Study the drawing (mm; zero at the part's minimum x, y, z) and answer. A direction names the side the tool comes from. Round coordinates to 2 decimals unless told otherwise and drop trailing zeros. Write each loop counter-clockwise with the first axis right and the second up, starting at its lowest first coordinate (ties: lowest second). Pieces come first, ordered by that corner, then holes. Notation, with made-up numbers: M 58.25,-30 L 78.25,-30 A21 ccw 78.25,-11 Z; hole C 52.5,54 d1. An arc over 180 degrees is marked long. Write each question's results on one line, items separated by ' | '.
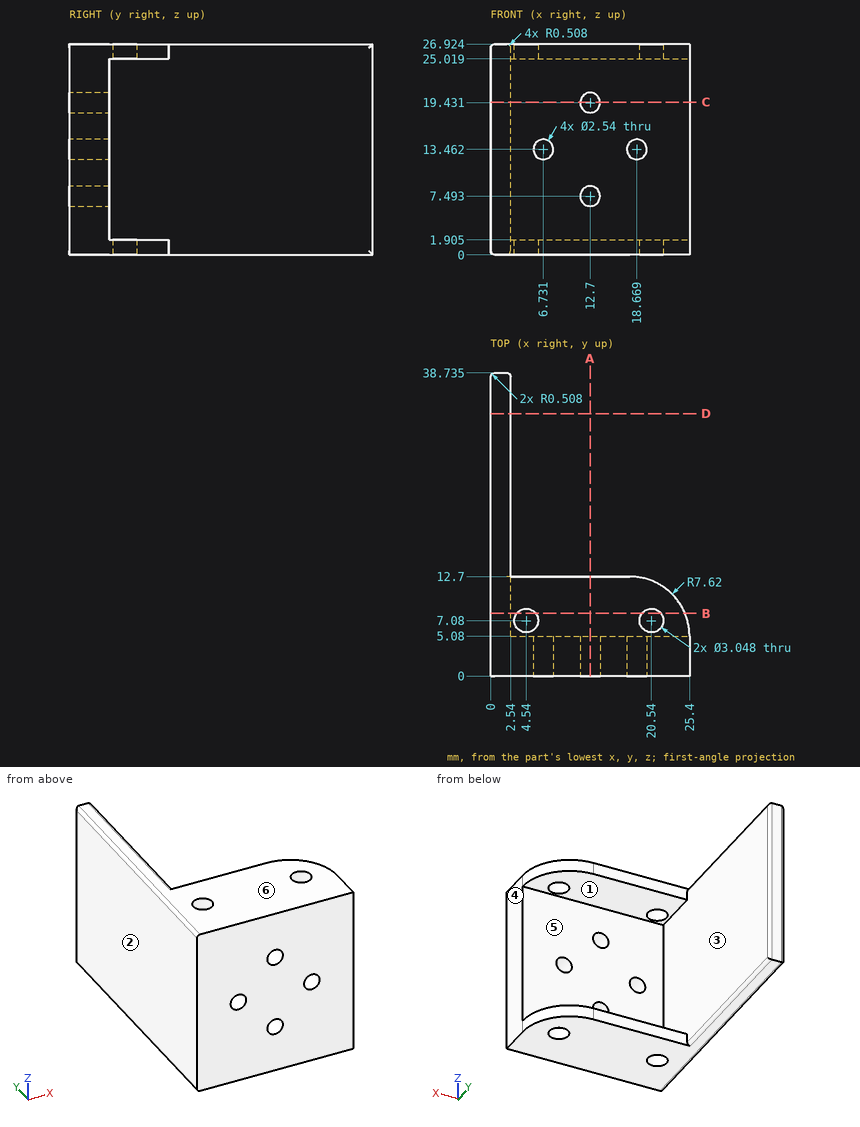
1) Section A-A (x = 12.7) is taken. Determine the outline of the cut face in (y, z) (3 decimals).
Return value:
outline: M 0,0 L 12.7,0 L 12.7,1.905 L 5.08,1.905 L 5.08,6.223 L 0,6.223 Z; M 0,8.763 L 5.08,8.763 L 5.08,18.161 L 0,18.161 Z; M 0,20.701 L 5.08,20.701 L 5.08,25.019 L 12.7,25.019 L 12.7,26.924 L 0,26.924 Z
2) Section C-C (z = 19.5) is taken. Determine the outline of the cut face in (x, y) (3 decimals), then the cut area to 3 significant figures.
Return value:
outline: M 0,0 L 11.432,0 L 11.432,5.08 L 2.54,5.08 L 2.54,38.227 A0.508 ccw 2.032,38.735 L 0.508,38.735 A0.508 ccw 0,38.227 Z; M 13.968,0 L 25.4,0 L 25.4,5.08 L 13.968,5.08 Z | area: 202 mm²
3) Each of these flat-tipped pins is pushed along its axis until it touches: pin 1 (12 mm diameter, centred on x = 13, z = 13.5, fed in from +Y); pin 2 (2 mm diameter, centred on x = 12, z = 0.5, fed in from +Y); pin 3 (2 mm diameter, centred on x = 18.669, z = 13.462, fed in from -Y); pin 4 (3 mm diameter, centred on y = 10, z = 7.5, fed in from +X). Where does it stop, or does it pass through?
Return value:
pin 1: y = 5.08 | pin 2: y = 12.7 | pin 3: through | pin 4: x = 2.54
4) Find the intervals of material crossed by line 1 (Z direction, x = 14.75, y = 11) (3 decimals); line 2 (Y direction, x = 20.54, z = 25.9); line 3 (Y direction, x = 13.5, z = 23.5), in increasing order.
Return value:
line 1: 0 to 1.905, 25.019 to 26.924 | line 2: 0 to 5.56, 8.6 to 12.18 | line 3: 0 to 5.08
5) The mould has two halves that part along Z. Classify the marked faces 3, 4, 5 and 6: +Z half, -Z half, draft (parallel to the pull), parting line (faces both ways), or undercut.
Return value:
face 3: undercut | face 4: draft | face 5: undercut | face 6: +Z half
6) Section D-D (y = 33.5) is taken. Determine the outline of the cut face in (x, z).
Return value:
outline: M 0,0.51 A0.51 ccw 0.51,0 L 2.03,0 A0.51 ccw 2.54,0.51 L 2.54,26.42 A0.51 ccw 2.03,26.92 L 0.51,26.92 A0.51 ccw 0,26.42 Z
7) Section B-B (y = 8) is taken. Determine the outline of the cut face in (x, z) (3 decimals), then the cut area to 3 significant figures.
Return value:
outline: M 0,0.508 A0.508 ccw 0.508,0 L 3.325,0 L 3.325,1.905 L 2.54,1.905 L 2.54,25.019 L 3.325,25.019 L 3.325,26.924 L 0.508,26.924 A0.508 ccw 0,26.416 Z; M 5.755,0 L 19.325,0 L 19.325,1.905 L 5.755,1.905 Z; M 5.755,25.019 L 19.325,25.019 L 19.325,26.924 L 5.755,26.924 Z; M 21.755,0 L 24.818,0 L 24.818,1.905 L 21.755,1.905 Z; M 21.755,25.019 L 24.818,25.019 L 24.818,26.924 L 21.755,26.924 Z | area: 135 mm²
8) A tool of negligible diameter and unlimited length cuts with its end or side. For the marked faces 1 and 2, from which of +Z, -Z, +X, -X, +Y, -Y can it reach the whole face along a straight path? Write none if from no direction.
Return value:
face 1: +X, +Y | face 2: +Z, -Z, -X, +Y, -Y
